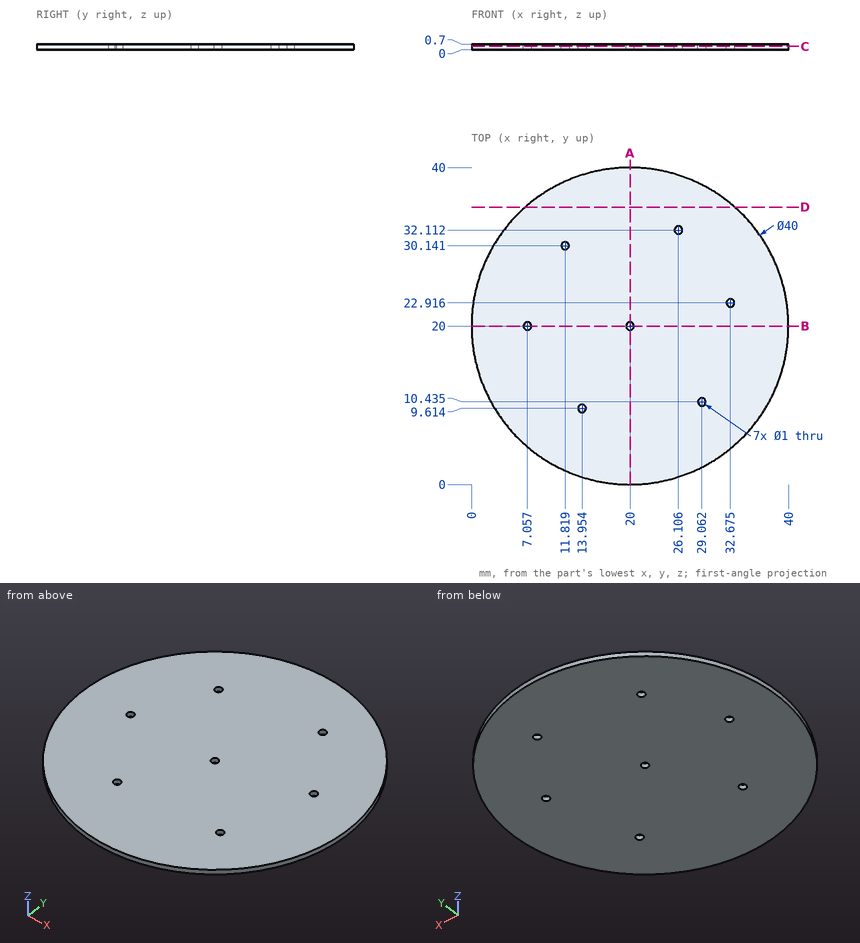
Job drawing, mm, ordinate dimensions from the low corner. One solid piece. Give positions to 0.01 mm unless a question says otherwise; leave off trailing zeros. Order: outer loops, then holes, each group sorted by start corner. A loop starts at its lowest first (then second) coordinate and runs counter-clockwise, first axis right, second up. Notation, with made-up numbers: (9, -7.5) -> (45, -7.5) arc R33 ccw to (45, 21.5) -> close; hole circle Ø3 at (71, 2.25). An arc over 180 degrees is marked (long way). Return JSON: item names as keys, results as strings.
Q1. Drill centre lines: line 1 (Y direction, x = 20, z = 0.35); line 2 (Y direction, x = 33, z = 0.25) (1 decimal); line 3 (X direction, y = 32.5, z = 0.1) (1 decimal). Where is each one in solid material? Low to high.
Working result:
{"line 1": "0 to 19.5, 20.5 to 40", "line 2": "4.8 to 22.5, 23.3 to 35.2", "line 3": "4.4 to 25.8, 26.4 to 35.6"}
Q2. Saw through at A-A (x = 20). Write the cut outline in (y, z).
Working result:
{"outline": "(0, 0) -> (19.5, 0) -> (19.5, 0.7) -> (0, 0.7) -> close; (20.5, 0) -> (40, 0) -> (40, 0.7) -> (20.5, 0.7) -> close"}
Q3. Saw through at D-D (y = 35). Write the cut outline in (x, z).
Working result:
{"outline": "(6.77, 0) -> (33.23, 0) -> (33.23, 0.7) -> (6.77, 0.7) -> close"}
Q4. Saw through at C-C (z = 0.4). Write the cut outline in (x, y) (1 decimal), then the cut area to 3 significant figures.
Working result:
{"outline": "circle Ø40 at (20, 20); hole circle Ø1 at (7.1, 20); hole circle Ø1 at (11.8, 30.1); hole circle Ø1 at (14, 9.6); hole circle Ø1 at (20, 20); hole circle Ø1 at (26.1, 32.1); hole circle Ø1 at (29.1, 10.4); hole circle Ø1 at (32.7, 22.9)", "area": "1,250 mm²"}
Q5. Saw through at B-B (y = 20). Write the cut outline in (x, z).
Working result:
{"outline": "(0, 0) -> (6.56, 0) -> (6.56, 0.7) -> (0, 0.7) -> close; (7.56, 0) -> (19.5, 0) -> (19.5, 0.7) -> (7.56, 0.7) -> close; (20.5, 0) -> (40, 0) -> (40, 0.7) -> (20.5, 0.7) -> close"}
